Read the model definition and answer for the solid it produces. Units are mm, in the model's axes. Give positions to 0.01 mm unless a question says otherwise; leave off trailing zeros. Write each loop counter-clockwise with the first axis right and the second up, starting at its lowest first coordinate (ties: lowest second). Pieces come first, ordered by that corner, then holes. Notation, with made-up numbers: (-39.5, -37) -> (8.5, -37) arc R30 ccw to (8.5, -10) -> close; hole circle Ø5 at (-37.75, 76.5). An arc over 180 degrees is marked (long way). Write item = value, one per line.
Autodesk Inventor part; units mm, degrees
ref_plane "Work Plane1" through (7.5, 0, 7.5) normal (0.7071, 0.7071, 0) x (0, 0, -1)
ref_plane "Work Plane2" through (-7.5, 0, 7.5) normal (0, 0.7071, 0.7071) x (1, 0, 0)
ref_plane "Work Plane3" through (-7.5, 0, -7.5) normal (0.7071, -0.7071, 0) x (0.5774, 0.5774, 0.5774)
sketch "Sketch1" plane through (0, 0, 0) normal (0, 1, 0) x (-1, 0, 0)
  line L0 (7.5, 7.5) -> (-7.5, 7.5)
  line L1 (-7.5, 7.5) -> (-7.5, -7.5)
  line L2 (-7.5, -7.5) -> (7.5, -7.5)
  line L3 (7.5, -7.5) -> (7.5, 7.5)
  line L4 (7.5, 7.5) -> (-7.5, -7.5) construction
  line L5 (-7.5, 7.5) -> (7.5, -7.5) construction
  point P0 (0, 0)
  dimension "d0" = 15
  dimension "d1" = 15
extrude "Extrusion1" add sketch "Sketch1" along normal blind 7.5
sketch "Sketch2" plane through (0, 7.5, 0) normal (0, 1, 0) x (1, 0, 0)
  point P0 (0, 0)
  point P1 (0, 0)
ref_plane "Work Plane1" through (7.5, 0, 7.5) normal (0.7071, 0.7071, 0) x (0, 0, -1)
ref_plane "Work Plane2" through (-7.5, 0, 7.5) normal (0, 0.7071, 0.7071) x (1, 0, 0)
ref_plane "Work Plane3" through (-7.5, 0, -7.5) normal (0.7071, -0.7071, 0) x (0.5774, 0.5774, 0.5774)
ref_plane "Work Plane4" through (7.5, 0, -7.5) normal (0, 0.7071, -0.7071) x (-1, 0, 0)
sketch "Sketch4" plane through (7.5, 0, 7.5) normal (0.7071, 0.7071, 0) x (0, 0, -1)
  line L0 (26.6476, 25.9998) -> (-15.2684, 25.9998)
  line L1 (-15.2684, 25.9998) -> (-15.2684, -13.1545)
  line L2 (-15.2684, -13.1545) -> (26.6476, -13.1545)
  line L3 (26.6476, -13.1545) -> (26.6476, 25.9998)
  point P0 (7.5, 5.3033)
extrude "Extrusion2" cut sketch "Sketch4" along normal through all
sketch "Sketch5" plane through (-7.5, 0, 7.5) normal (0, 0.7071, 0.7071) x (1, 0, 0)
  line L0 (25.5392, 33.5657) -> (-14.5967, 33.5657)
  line L1 (-14.5967, 33.5657) -> (-14.5967, -23.0742)
  line L2 (-14.5967, -23.0742) -> (25.5392, -23.0742)
  line L3 (25.5392, -23.0742) -> (25.5392, 33.5657)
  point P0 (7.5, 5.3033)
extrude "Extrusion3" cut sketch "Sketch5" along normal through all
sketch "Sketch6" plane through (-7.5, 0, -7.5) normal (0.7071, -0.7071, 0) x (0.5774, 0.5774, 0.5774)
  line L0 (35.4927, -22.9081) -> (-17.0623, -22.9081)
  line L1 (-17.0623, -22.9081) -> (-17.0623, 39.3429)
  line L2 (-17.0623, 39.3429) -> (35.4927, 39.3429)
  line L3 (35.4927, 39.3429) -> (35.4927, -22.9081)
  point P0 (8.6603, 3.0619)
extrude "Extrusion4" cut sketch "Sketch6" against normal blind 15
sketch "Sketch7" plane through (7.5, 0, -7.5) normal (0, 0.7071, -0.7071) x (-1, 0, 0)
  line L0 (-15.9671, 26.9617) -> (32.6533, 26.9617)
  line L1 (32.6533, 26.9617) -> (32.6533, -21.7992)
  line L2 (32.6533, -21.7992) -> (-15.9671, -21.7992)
  line L3 (-15.9671, -21.7992) -> (-15.9671, 26.9617)
  point P0 (7.5, 5.3033)
extrude "Extrusion5" cut sketch "Sketch7" along normal through all
equation "\"d0\" = 0.5 * BodyHeight"
equation "\"d1\" = 0.5 * BodyHeight"
equation "\"d2\" = 0.25 * BodyHeight"
equation "\"d8\" = 0.5 * BodyHeight"
properties part number "HexSideSpike" material "H TPU"
(1) Given P1, Ø1.5, axis at y = 4, z = -1, coming from the +X side; P2, Ø4, axis at x = 3.5, z = 3, coming from the +Y side; P3, Ø4, axis at y = 3.5, z = 3, coming from the +X side, each flat-ended and moving along its own axis, determine where each tip first touches the part or whether it passes through.
Checks:
P1 = 4.25
P2 = 5.64
P3 = 6
(2) The part is cut by section A-A on x = 5.25. Determine the outline of the cut face in (y, z), plus the area to 3 significant figures.
Checks:
outline = (0, -7.5) -> (2.25, -5.25) -> (2.25, 5.25) -> (0, 7.5) -> close
area = 28.7 mm²
(3) Consider L1, parallel to X at y = 3.75, z = -3; L2, parallel to Y at x = 4, z = -6; L3, parallel to Z at x = 3.5, y = 1.25. Determine where each line is inside the solid, lowest interval first.
Checks:
L1 = -3.75 to 3.75
L2 = 0 to 1.5
L3 = -6.25 to 6.25
(4) The part is cut by section B-B on z = 0.5. Determine the outline of the cut face in (x, y).
Checks:
outline = (-7.5, 0) -> (7.5, 0) -> (0.5, 7) -> (-0.5, 7) -> close
